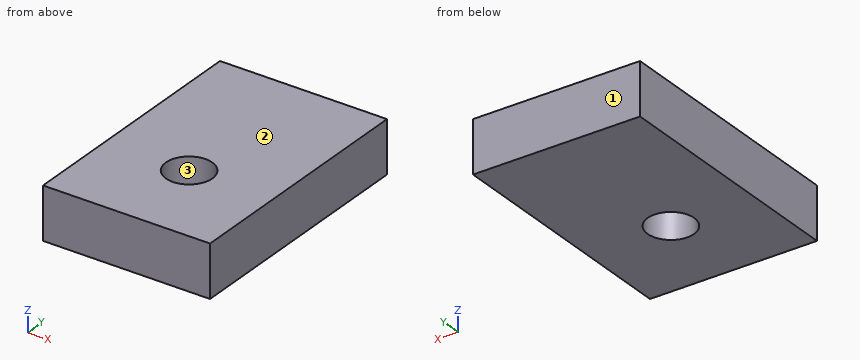
```python
from build123d import *

# Parameters (mm, degrees)
CYLINDER1615_R     = 4
CYLINDER1615_DEPTH = 100
BOX641_W           = 28.8
BOX641_H           = 43.38
BOX641_DEPTH       = 9


with BuildPart() as obj1:
    # Cylinder1615 → Cylinder1615 (new body)
    with BuildSketch(Plane.XY):
        Circle(CYLINDER1615_R)
    extrude(amount=CYLINDER1615_DEPTH)


with BuildPart() as cut307:
    # Box641 → Box641 (new body)
    with BuildSketch(Plane(origin=(-14.4, -15.34, 34), x_dir=(1, 0, 0), z_dir=(0, 0, 1))):
        with Locations((14.4, 21.69)):
            Rectangle(BOX641_W, BOX641_H)
    extrude(amount=BOX641_DEPTH)

    # Cut307: cut obj1
    add(obj1.part, mode=Mode.SUBTRACT)


with BuildPart() as cut307_1:
    # Cut307 placement: moved
    add(cut307.part.moved(Location((0, 90, -86))))


solid = cut307_1.part
```
Geometry: final body of the model. Coordinates: model frame, mm. Face numbers are marked on the shaded views. Give positions to 0.01 mm unless a question says otherwise; leave off trailing zeros. Loops run counter-clockwise (first coordinate to the right, second up) from the corner with the lowest first, then second, coordinate; pieces in that order, holes last. Notation, with made-up numbers: (-13, 27) - (29, 27) arc R36 ccw to (29, 61) - close; hole circle Ø11 at (64.5, -39.75). An arc over 180 degrees is marked (long way). Answer as CSV lines item,"result". Start each with the question number.
(1) Section query A-A (y = 90). Output: boundary loops of the cut face in (x, z).
(2) Section query C-C (z = -44.5). Output: boundary loops of the cut face in (x, y).
(3) Ray query, line 1 along X through (y, z) = (90, -46.5); line 2 along Y through (x, z) = (0, -48.5); line 3 along X through (y, z) = (89, -43.5). Return the intervals inside material, ascending. Write a range as [from, to].
(4) Mould query, pull axis Y, two halves, no side actions, for the marked faces 1, 2 and 3. Classes: +Y half, -Y half, draft (parallel to the pull), parting line (faces both ways), or undercut.
(5) Section query B-B (x = 0). Output: boundary loops of the cut face in (y, z), and give its area (3 significant figures).
Worked answers:
1,outline,"(-14.4, -52) - (-4, -52) - (-4, -43) - (-14.4, -43) - close; (4, -52) - (14.4, -52) - (14.4, -43) - (4, -43) - close"
2,outline,"(-14.4, 74.66) - (14.4, 74.66) - (14.4, 118.04) - (-14.4, 118.04) - close; hole circle Ø8 at (0, 90)"
3,line 1,"x = [-14.4, -4], [4, 14.4]"
3,line 2,"y = [74.66, 86], [94, 118.04]"
3,line 3,"x = [-14.4, -3.87], [3.87, 14.4]"
4,face 1,"+Y half"
4,face 2,"draft"
4,face 3,"undercut"
5,outline,"(74.66, -52) - (86, -52) - (86, -43) - (74.66, -43) - close; (94, -52) - (118.04, -52) - (118.04, -43) - (94, -43) - close"
5,area,"318 mm^2"
